```python
from build123d import *

# Parameters (mm, degrees)
SKETCH_1_W                  = 22
SKETCH_1_H                  = 40
EXTRUDE_1_DEPTH             = 11
SKETCH_4_R                  = 1.6
CUT_EXTRUDE_3_DEPTH         = 12
PATTERN_LINEAR_1_COUNT      = 2
PATTERN_LINEAR_1_PITCH      = 14
PATTERN_LINEAR_1_COUNT_DIR2 = 2
PATTERN_LINEAR_1_PITCH_DIR2 = 15
CHAMFER_1_SIZE              = 2


with BuildPart() as part:
    # 草圖1 → 填料-伸長1 (new body)
    with BuildSketch(Plane.XY):
        Rectangle(SKETCH_1_W, SKETCH_1_H)
    extrude(amount=EXTRUDE_1_DEPTH)

    # 草圖4 → 除料-伸長3 (cut, through all)
    with BuildSketch(Plane.XY.offset(11)):
        with Locations((-7, 7.5)):
            Circle(SKETCH_4_R)
    cut_extrude_3 = extrude(amount=-CUT_EXTRUDE_3_DEPTH, mode=Mode.SUBTRACT)

    # 直線複製排列1: Cut-Extrude 3 2 × 2
    with Locations(*[(i * PATTERN_LINEAR_1_PITCH, -j * PATTERN_LINEAR_1_PITCH_DIR2, 0) for i in range(PATTERN_LINEAR_1_COUNT) for j in range(PATTERN_LINEAR_1_COUNT_DIR2) if (i, j) != (0, 0)]):
        add(cut_extrude_3, mode=Mode.SUBTRACT)

    # 導角1
    chamfer_1_edges = [part.edges().sort_by_distance(p)[0] for p in [
        (11, -20, 5.5),
        (-11, -20, 5.5),
        (-11, 20, 5.5),
        (11, 20, 5.5),
    ]]
    chamfer(chamfer_1_edges, length=CHAMFER_1_SIZE)


solid = part.part
```
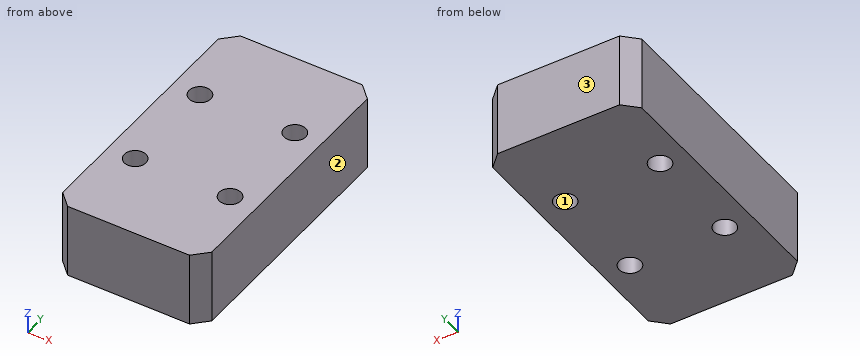
Input: part model. Units: mm. Frame: model coordinates. Face numbers are marked on the shaded views. Coordinates: 2 decimals unless noted, no trailing zeros. Write each loop counter-clockwise with the first axis right and the second up, starting at its lowest first coordinate (ties: lowest second). Pieces come first, ordered by that corner, then holes.
1) Material intervals for line 1 along Y through (x, z) = (7, 6.25); line 2 along X through (y, z) = (-7, 8.5); line 3 along Y through (x, z) = (8, 5.5), sorted ascending.
2) Section A-A on x = 7. Output: boundary loops of the cut face in (y, z), and give its area (3 significant figures).
3) Pin query (flat end, axial travel): pin 1 Ø3.5 at (x, y) = (-7, -7.5) entering from +Z; pin 2 Ø2.5 at (x, y) = (-7, 7.5) entering from +Z. Return the tip coordinate at first contact, or that it passes through.
4) Section B-B on z = 6.5. Output: boundary loops of the cut face in (x, y), and give its area (3 significant figures).
5) Mould query, pull axis X, two halves, no side actions, for the marked faces 1, 2 and 3. Classes: pulls with the +X half, pulls with the -X half, needs draft (parallel to the pull), parting line crosses it, or undercut.
6) Section C-C on y = -7.5. Output: boundary loops of the cut face in (x, z).
7) Section D-D on x = 9.75. Output: boundary loops of the cut face in (y, z), and give its area (4 significant figures).
Check result:
1. line 1: y = -20 to -9.1, -5.9 to 5.9, 9.1 to 20
1. line 2: x = -11 to -8.52, -5.48 to 5.48, 8.52 to 11
1. line 3: y = -20 to -8.75, -6.25 to 6.25, 8.75 to 20
2. outline: (-20, 0) - (-9.1, 0) - (-9.1, 11) - (-20, 11) - close; (-5.9, 0) - (5.9, 0) - (5.9, 11) - (-5.9, 11) - close; (9.1, 0) - (20, 0) - (20, 11) - (9.1, 11) - close
2. area: 370 mm2
3. pin 1: stops at z = 11
3. pin 2: passes through
4. outline: (-11, -18) - (-9, -20) - (9, -20) - (11, -18) - (11, 18) - (9, 20) - (-9, 20) - (-11, 18) - close; hole circle Ø3.2 at (-7, -7.5); hole circle Ø3.2 at (-7, 7.5); hole circle Ø3.2 at (7, -7.5); hole circle Ø3.2 at (7, 7.5)
4. area: 840 mm2
5. face 1: undercut
5. face 2: pulls with the +X half
5. face 3: needs draft
6. outline: (-11, 0) - (-8.6, 0) - (-8.6, 11) - (-11, 11) - close; (-5.4, 0) - (5.4, 0) - (5.4, 11) - (-5.4, 11) - close; (8.6, 0) - (11, 0) - (11, 11) - (8.6, 11) - close
7. outline: (-19.25, 0) - (19.25, 0) - (19.25, 11) - (-19.25, 11) - close
7. area: 423.5 mm2
